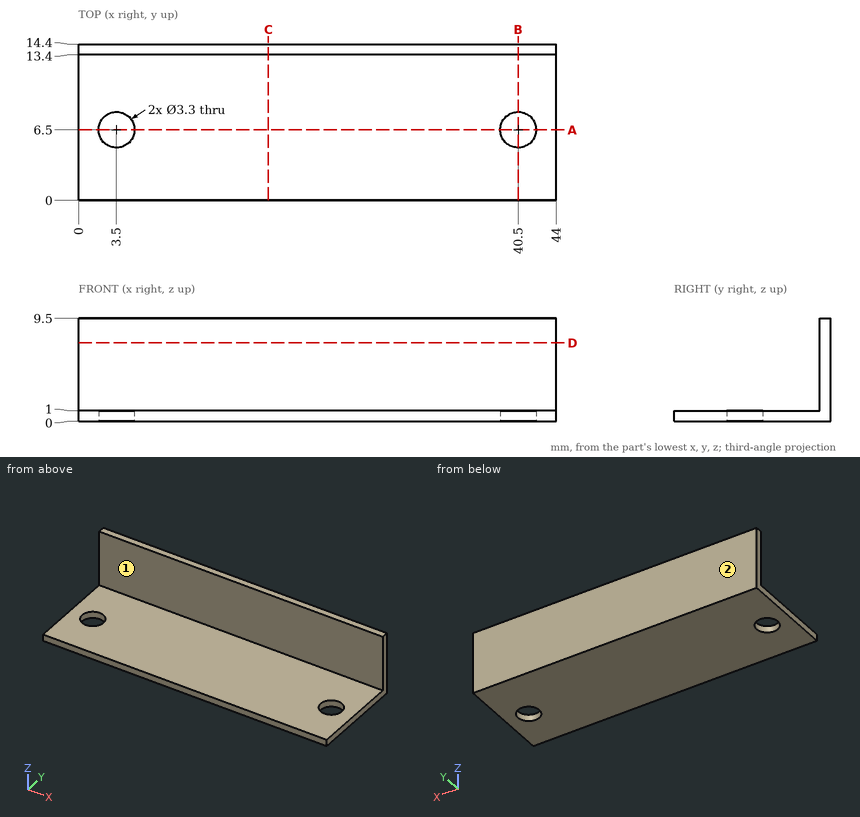
Check sheet for the drawn part. Datum: minimum x, y, z corner. Units: mm. A direction names the side the tool comes from. Give positions to 0.01 mm unless a question says otherwise; leave off trailing zeros. Write each loop counter-clockwise with the first axis right and the second up, starting at its lowest first coordinate (ties: lowest second). Pieces come first, ordered by that corner, then holes. Notation, with made-up numbers: M 83.5,12.5 L 134.5,12.5 A28 ccw 134.5,31.5 Z; hole C -39,-36.5 d6. An arc over 180 degrees is marked long. Write item = value, one per line.
(1) Sectioned sample at B-B (x = 40.5). Record the cut outline in (y, z), then the cut area to 3 significant figures.
Found:
outline = M 0,0 L 4.85,0 L 4.85,1 L 0,1 Z; M 8.15,0 L 14.4,0 L 14.4,9.5 L 13.4,9.5 L 13.4,1 L 8.15,1 Z
area = 19.6 mm2
(2) Sectioned sample at A-A (y = 6.5). Record the cut outline in (x, z).
Found:
outline = M 0,0 L 1.85,0 L 1.85,1 L 0,1 Z; M 5.15,0 L 38.85,0 L 38.85,1 L 5.15,1 Z; M 42.15,0 L 44,0 L 44,1 L 42.15,1 Z
(3) Sectioned sample at C-C (x = 17.5). Record the cut outline in (y, z).
Found:
outline = M 0,0 L 14.4,0 L 14.4,9.5 L 13.4,9.5 L 13.4,1 L 0,1 Z
(4) Access from +Z, -Z, +X, -X, +Y, -Y to the whole of each face (thin tool, end or side, straight path). Record for the marked faces 1 and 2.
Found:
face_1 = +Z, +X, -X, -Y
face_2 = +Z, -Z, +X, -X, +Y
(5) Material ranges on line 1 (Y direction, x = 40.5, z = 0.3); line 2 (Y direction, x = 38, z = 4); line 3 (X direction, y = 5, z = 0.75), recorded low to high.
Found:
line_1 = 0 to 4.85, 8.15 to 14.4
line_2 = 13.4 to 14.4
line_3 = 0 to 2.81, 4.19 to 39.81, 41.19 to 44
(6) Sectioned sample at D-D (z = 7.25). Record the cut outline in (x, y).
Found:
outline = M 0,13.4 L 44,13.4 L 44,14.4 L 0,14.4 Z
(7) Go/stop test with flat-tipped pins: pin 1 Ø6 at (x, y) = (24.5, 8) entering from +Z; pin 2 Ø2.5 at (x, y) = (3.5, 6.5) entering from -Z; pin 3 Ø1 at (x, z) = (6, 3.5) entering from -Y. Record where each tip stops, or that it passes through.
Found:
pin_1 = 1
pin_2 = through
pin_3 = 13.4
